Input: part model. Units: mm. Frame: model coordinates. Face numbers are marked on the shaded views. Coordinates: 2 decimals unless noted, no trailing zeros.
1) Draft query along Z for the marked faces 1 and 2. Return one class per face: pulls with the +Z half, pulls with the -Z half, needs draft (parallel to the pull), parting line crosses it, or undercut.
2) Section query A-A (z = 0). State how many separate pieces and enclosed holes the cut face has, then the cut area to 3 significant figures.
3) Pin query (flat end, axial travel): pin 1 Ø4 at (y, z) = (-53.975, 0) entering from +X; pin 2 Ø3 at (x, z) = (-4, -17.5) entering from +Y; pin 3 Ø2 at (y, z) = (45.5, 4.5) entering from -X; pin 4 Ø2 at (x, z) = (1.5, 40.5) entering from -Y. Return the tip coordinate at first contact, or that it passes through.
4) Line query: L1, parallel to Y at x = 4.25, z = 0 (3 decimals); L2, parallel to Z at x = 1, y = 38; L3, parallel to X at y = -33.5, z = -10. Output: solid intervals per line, ascending.
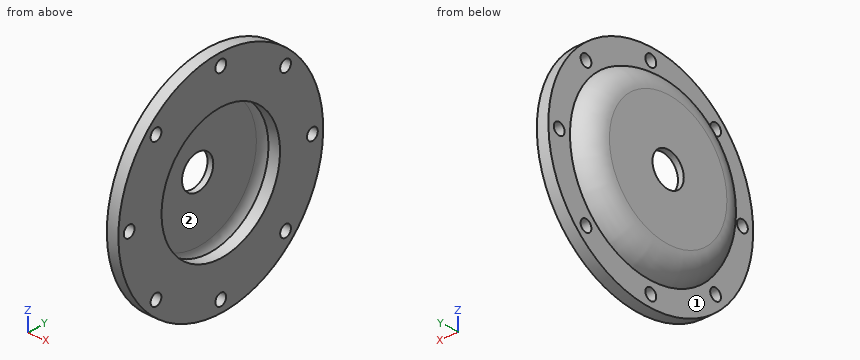
from build123d import *

# Parameters (mm, degrees)
SKETCH2_W               = 6.35
SKETCH2_H               = 25.4
CUT_EXTRUDE1_DEPTH      = 86.84251205
CUT_EXTRUDE1_DEPTH_BACK = 86.84251205
SKETCH3_R               = 3.175


with BuildPart() as part:
    # Sketch2 → Revolve1 (revolve)
    with BuildSketch(Plane.XY, mode=Mode.PRIVATE) as revolve1_sk:
        with BuildLine():
            ThreePointArc((-6.35, 34.6075), (-4.624734672, 40.464062692), (0, 44.45))
            Line((0, 44.45), (0, 47.625))
            ThreePointArc((0, 47.625), (-6.88946039, 42.67256248), (-9.525, 34.6075))
            Line((-9.525, 34.6075), (-9.525, 9.2075))
            Line((-9.525, 9.2075), (-6.35, 9.2075))
            Line((-6.35, 9.2075), (-6.35, 34.6075))
        make_face()
        with Locations((3.175, 47.625)):
            Rectangle(SKETCH2_W, SKETCH2_H)
    revolve(revolve1_sk.sketch.rotate(Axis((-978.527794003, 0, 0), (1, 0, 0)), 90), axis=Axis((-978.527794003, 0, 0), (1, 0, 0)))

    # Sketch3 → Cut-Extrude1 (cut, two sides: drawn at the far end of the back side and taken through both)
    with BuildSketch(Plane.ZY.offset(-CUT_EXTRUDE1_DEPTH_BACK)):
        with Locations((0, 53.975)):
            Circle(SKETCH3_R)
        with Locations((38.166088515, 38.166088515)):
            Circle(SKETCH3_R)
        with Locations((53.975, 0)):
            Circle(SKETCH3_R)
        with Locations((38.166088515, -38.166088515)):
            Circle(SKETCH3_R)
        with Locations((0, -53.975)):
            Circle(SKETCH3_R)
        with Locations((-38.166088515, -38.166088515)):
            Circle(SKETCH3_R)
        with Locations((-53.975, 0)):
            Circle(SKETCH3_R)
        with Locations((-38.166088515, 38.166088515)):
            Circle(SKETCH3_R)
    extrude(amount=CUT_EXTRUDE1_DEPTH + CUT_EXTRUDE1_DEPTH_BACK, mode=Mode.SUBTRACT)


solid = part.part
Answer:
1. face 1: needs draft
1. face 2: undercut
2. separate pieces: 4
2. enclosed holes: 0
2. area: 495 mm2
3. pin 1: passes through
3. pin 2: stops at y = 43.31
3. pin 3: stops at x = -5.05
3. pin 4: stops at y = -45.59
4. L1: y = -60.325 to -57.15, -50.8 to -34.925, 34.925 to 50.8, 57.15 to 60.325
4. L2: z = -46.85 to -41.34, -35 to 35, 41.34 to 46.85
4. L3: x = -9.52 to -6.34, 0 to 6.35
